Verification items for the finished model (mm, model axes). A direction names the side the tool comes from. Give positions to 0.01 mm unless a question says otherwise; leave off trailing zeros. Write each loop counter-clockwise with the first axis right and the second up, starting at its lowest first coordinate (ties: lowest second). Pieces come first, ordered by that corner, then holes.
Autodesk Inventor part; units mm, degrees
ref_plane "YZ Plane" through (0, 0, 0) normal (1, 0, 0) x (0, 1, 0)
ref_plane "XZ Plane" through (0, 0, 0) normal (0, 1, 0) x (-1, 0, 0)
ref_plane "XY Plane" through (0, 0, 0) normal (0, 0, 1) x (1, 0, 0)
sketch "スケッチ1" plane through (0, 0, 0) normal (0, 1, 0) x (-1, 0, 0)
  circle A0 centre (0, 0) radius 10
  line L0 (0, 10) -> (-10, 10)
  line L1 (-10, 10) -> (-10, -10)
  line L2 (-10, -10) -> (10, -10)
  line L3 (10, -10) -> (10, 0)
  dimension "d0" = 20
  dimension "d1" = 10
  dimension "d2" = 10
extrude "押し出し1" add sketch "スケッチ1" along normal blind 77
sketch "スケッチ2" plane through (0, 0, 10) normal (0, 0, 1) x (1, 0, 0)
  line L0 (0, 0) -> (0, 77)
  line L1 (0, 77) -> (10, 77)
  line L2 (10, 77) -> (10, 0)
  line L3 (10, 0) -> (0, 0)
extrude "押し出し2" cut sketch "スケッチ2" against normal blind 1
sketch "スケッチ3" plane through (-10, 0, -10) normal (-1, 0, 0) x (0, 0, 1)
  line L0 (0, 77) -> (10, 77)
  line L1 (10, 0) -> (10, 77)
  line L2 (10, 0) -> (0, 0)
  line L3 (0, 0) -> (0, 77)
extrude "押し出し3" cut sketch "スケッチ3" against normal blind 1
sketch "スケッチ4" plane through (0, 0, 9) normal (0, 0, 1) x (1, 0, 0)
  line L0 (0, 77) -> (10, 77)
  line L1 (10, 77) -> (10, 0)
  line L2 (10, 0) -> (0, 0)
  point P0 (5, 72)
  point P1 (5, 5)
  dimension "d9" = 5
  dimension "d10" = 5
  dimension "d11" = 5
hole "穴1" at (5, 72, 9) at (5, 5, 9) direction (0, 0, -1) diameter 5 depth 6 tip angle 118
sketch "スケッチ5" plane through (0, 0, 0) normal (0, 1, 0) x (1, 0, 0)
  point P0 (0, 0)
hole "穴2" at (0, 0, 0) direction (0, 1, 0) diameter 5 depth 6 tip angle 118
sketch "スケッチ6" plane through (-9, 0, -10) normal (-1, 0, 0) x (0, 0, 1)
  line L0 (0, 0) -> (0, 77)
  line L1 (0, 77) -> (10, 77)
  line L2 (10, 0) -> (0, 0)
  point P0 (5, 72)
  point P1 (5, 5)
  dimension "d26" = 5
  dimension "d27" = 5
  dimension "d28" = 5
  dimension "d29" = 5
hole "穴3" at (-9, 72, -5) at (-9, 5, -5) direction (1, 0, 0) diameter 5 depth 6 tip angle 118
sketch "スケッチ7" plane through (0, 77, 0) normal (0, 1, 0) x (1, 0, 0)
  circle A0 centre (0, 0) radius 3.05
  dimension "d37" = 6.1
extrude "押し出し4" cut sketch "スケッチ7" against normal blind 6
chamfer "面取り1" distance 3 angle 45 1 edges at (-3.05, 77, 0)
fillet "フィレット1" radius 10 1 edges at (10, 38.5, -10)
properties part number "base6" material "ABS プラスチック"
Item 1: Scan lines: line 1 along Y through (x, z) = (-4.65, -5); line 2 along Y through (x, z) = (7, 5.25); line 3 along Z through (x, y) = (-6.35, 5). Record each from-to range of solid material in increasing order.
Answer key:
line 1: y = 0 to 2.5, 7.5 to 69.5, 74.5 to 77
line 2: y = 0 to 3.5, 6.5 to 70.5, 73.5 to 77
line 3: z = -10 to -7.5, -2.5 to 7.73
Item 2: Set-up check for faces 1 (the face through (-9, 39, -5)), 2 (the face through (2.44, 3.04, 0.54)), 3 (the face through (4.9, 74.5, 6)), 4 (the face through (-3.047, 72.521, -0.134)), 5 (the face through (-5.958, 4.249, -2.615)): record each of +Z, -Z, +X, -X, +Y, -Y from which the full face is reachable in a straight line by a thin tool's end or side.
Answer key:
face 1: -Z, -X, +Y, -Y
face 2: -Y
face 3: +Z
face 4: +Y
face 5: -X
Item 3: Sectioned sample at B-B on x = -4.25. State how many separate pieces and enclosed holes the cut face has, then the cut area to 3 significant figures.
Answer key:
separate pieces: 1
enclosed holes: 2
area: 1,420 mm2
Item 4: Release check for a two-part mould opening along Y. For faces 6 (the face through (-2, 0, -2)), 7 (the face through (4.736, 72.345, 1.759)), 8 (the face through (0, 71, 0)) record: released by +Y, released by -Y, zero draft, split by the parting line, or undercut.
Answer key:
face 6: released by -Y
face 7: undercut
face 8: released by +Y
Item 5: Depth check by flat-ended pin: pin 1 (3 mm diameter, centred on x = 5, y = 72, fed in from -Z); pin 2 (4.5 mm diameter, centred on y = 5, z = -5, fed in from -X); pin 3 (6 mm diameter, centred on y = 72, z = -5, fed in from -X). Enter the tip coordinate at first touch or a pass-through.
Answer key:
pin 1: stops at z = -9.37
pin 2: stops at x = -2.85
pin 3: stops at x = -9
Item 6: Sectioned sample at A-A on y = 29. Record the cut outline in (x, z), then the cut area to 3 significant figures.
Answer key:
outline: (-10, 0) - (-9, 0) - (-9, -10) - (0, -10) arc R10 ccw to (10, 0) - (10, 9) - (0, 9) - (0, 10) arc R10 ccw to start
area: 337 mm2
